Read the model definition and answer for the solid it produces. Units are mm, in the model's axes. Coordinates: 2 decimals unless noted, no trailing zeros. Order: outer loops, then holes, each group sorted by start corner. A loop starts at its lowest first (then second) coordinate and runs counter-clockwise, first axis right, second up. Notation, with made-up numbers: M 12,-25 L 22,-25 A26 cw 22,12 Z; hole C 68.5,36 d8. An arc over 180 degrees is marked long. Put each result on its own line as item: value.
from build123d import *

# Parameters (mm, degrees)
SKETCH1_R           = 13
BOSS_EXTRUDE1_DEPTH = 5.5
FILLET2_R           = 3


with BuildPart() as part:
    # Sketch1 → Boss-Extrude1 (new, symmetric)
    with BuildSketch(Plane.XY):
        with BuildLine():
            Line((-15, -9.949874371), (-15, -209.949874371))
            Line((-15, -209.949874371), (15, -209.949874371))
            Line((15, -209.949874371), (15, -9.949874371))
            ThreePointArc((15, -9.949874371), (0, 18), (-15, -9.949874371))
        make_face()
        Circle(SKETCH1_R, mode=Mode.SUBTRACT)
    extrude(amount=BOSS_EXTRUDE1_DEPTH, both=True)

    # Fillet2
    # the kernel refuses this fillet: 3 mm, written as the material it adds along each edge
    with BuildSketch(Plane(origin=(15, -9.949874371, 5.5), x_dir=(0.5340574779916704, 0.8454481712093158, 0), z_dir=(0, 0, -1))) as fillet2_piece_1:
        with BuildLine():
            CenterArc((0.869355329, 2.999254564), FILLET2_R, 237.719985552, 31.002719134)
            Line((-0.732817105, 0.46291005), (0, 0))
            ThreePointArc((0, 0), (0.401240921, 0.004472619), (0.802481842, 0))
        make_face()
    extrude(amount=11)
    with BuildSketch(Plane(origin=(-15, -9.949874371, 5.5), x_dir=(0, -1, 0), z_dir=(0, 0, -1))) as fillet2_piece_2:
        with BuildLine():
            CenterArc((0.866779455, 3), FILLET2_R, 238.997280866, 31.002719134)
            ThreePointArc((-0.678456806, 0.428571429), (-0.336839767, 0.218067082), (0, 0))
            Line((0, 0), (0.866779455, 0))
        make_face()
    extrude(amount=11)
    # the kernel refuses this fillet: 3 mm, written as the material it takes off along each edge
    with BuildSketch(Plane(origin=(0, 0, -5.5), x_dir=(1, 0, 0), z_dir=(0, -1, 0))) as fillet2_2_piece_1:
        with BuildLine():
            CenterArc((13 + FILLET2_R, FILLET2_R), FILLET2_R, 180, 90)
            Line((13, FILLET2_R), (13, 0))
            Line((13, 0), (13 + FILLET2_R, 0))
        make_face()
    revolve(axis=Axis((0, 0, -5.5), (0, 0, 1)), mode=Mode.SUBTRACT)
    with BuildSketch(Plane(origin=(0, 0, 5.5), x_dir=(1, 0, 0), z_dir=(0, -1, 0))) as fillet2_2_piece_2:
        with BuildLine():
            CenterArc((13 + FILLET2_R, -FILLET2_R), FILLET2_R, 90, 90)
            Line((13, -FILLET2_R), (13, 0))
            Line((13, 0), (13 + FILLET2_R, 0))
        make_face()
    revolve(axis=Axis((0, 0, 5.5), (0, 0, 1)), mode=Mode.SUBTRACT)
    with BuildSketch(Plane(origin=(-22.5, -209.949874371, 5.5), x_dir=(0, 1, 0), z_dir=(1, 0, 0)), Plane(origin=(-22.5, -209.949874371, -5.5), x_dir=(0, 0, 1), z_dir=(1, 0, 0))) as fillet2_2_piece_3:
        with BuildLine():
            CenterArc((FILLET2_R, -FILLET2_R), FILLET2_R, 90, 90)
            Line((0, -FILLET2_R), (0, 0))
            Line((0, 0), (FILLET2_R, 0))
        make_face()
    extrude(amount=45, mode=Mode.SUBTRACT)
    with BuildSketch(Plane(origin=(15, -209.949874371, -13), x_dir=(-1, 0, 0), z_dir=(0, 0, 1)), Plane(origin=(-15, -209.949874371, -13), x_dir=(0, 1, 0), z_dir=(0, 0, 1))) as fillet2_2_piece_4:
        with BuildLine():
            CenterArc((FILLET2_R, -FILLET2_R), FILLET2_R, 90, 90)
            Line((0, -FILLET2_R), (0, 0))
            Line((0, 0), (FILLET2_R, 0))
        make_face()
    extrude(amount=26, mode=Mode.SUBTRACT)
    # the kernel refuses this fillet: 3 mm, written as the material it takes off along each edge
    with BuildSketch(Plane(origin=(-12, -206.949874371, 2.5), x_dir=(0, 0, 1), z_dir=(-1, 0, 0))) as fillet2_3_piece_1_section:
        Polygon((0, 0), (FILLET2_R, 0), (FILLET2_R, -FILLET2_R), (0, -FILLET2_R), align=None)
    fillet2_3_piece_1 = extrude(amount=FILLET2_R, mode=Mode.PRIVATE)
    fillet2_3_piece_1 = fillet2_3_piece_1 - Plane(origin=(-12, -206.949874371, 2.5), x_dir=(0, 0.7071067811865475, -0.7071067811865475), z_dir=(-1, 0, 0)) * Sphere(FILLET2_R, mode=Mode.PRIVATE)
    add(fillet2_3_piece_1, mode=Mode.SUBTRACT)
    with BuildSketch(Plane(origin=(-12, -206.949874371, -2.5), x_dir=(0, 0, -1), z_dir=(-1, 0, 0))) as fillet2_3_piece_2_section:
        Polygon((0, 0), (FILLET2_R, 0), (FILLET2_R, FILLET2_R), (0, FILLET2_R), align=None)
    fillet2_3_piece_2 = extrude(amount=FILLET2_R, mode=Mode.PRIVATE)
    fillet2_3_piece_2 = fillet2_3_piece_2 - Plane(origin=(-12, -206.949874371, -2.5), x_dir=(0, 0.7071067811865475, 0.7071067811865475), z_dir=(-1, 0, 0)) * Sphere(FILLET2_R, mode=Mode.PRIVATE)
    add(fillet2_3_piece_2, mode=Mode.SUBTRACT)
    with BuildSketch(Plane(origin=(12, -206.949874371, -2.5), x_dir=(1, 0, 0), z_dir=(0, 0, -1))) as fillet2_3_piece_3_section:
        Polygon((0, 0), (FILLET2_R, 0), (FILLET2_R, FILLET2_R), (0, FILLET2_R), align=None)
    fillet2_3_piece_3 = extrude(amount=FILLET2_R, mode=Mode.PRIVATE)
    fillet2_3_piece_3 = fillet2_3_piece_3 - Plane(origin=(12, -206.949874371, -2.5), x_dir=(-0.7071067811865475, 0.7071067811865475, 0), z_dir=(0, 0, -1)) * Sphere(FILLET2_R, mode=Mode.PRIVATE)
    add(fillet2_3_piece_3, mode=Mode.SUBTRACT)
    with BuildSketch(Plane(origin=(12, -206.949874371, 2.5), x_dir=(1, 0, 0), z_dir=(0, 0, 1))) as fillet2_3_piece_4_section:
        Polygon((0, 0), (FILLET2_R, 0), (FILLET2_R, -FILLET2_R), (0, -FILLET2_R), align=None)
    fillet2_3_piece_4 = extrude(amount=FILLET2_R, mode=Mode.PRIVATE)
    fillet2_3_piece_4 = fillet2_3_piece_4 - Plane(origin=(12, -206.949874371, 2.5), x_dir=(-0.7071067811865475, 0.7071067811865475, 0), z_dir=(0, 0, 1)) * Sphere(FILLET2_R, mode=Mode.PRIVATE)
    add(fillet2_3_piece_4, mode=Mode.SUBTRACT)
    with BuildSketch(Plane(origin=(15, -206.949874371, 5.5), x_dir=(-1, 0, 0), z_dir=(0, 1, 0)), Plane(origin=(-15, -10.816653826, -5.5), x_dir=(0, 0, 1), z_dir=(0, -1, 0))) as fillet2_3_piece_5:
        with BuildLine():
            CenterArc((FILLET2_R, -FILLET2_R), FILLET2_R, 90, 90)
            Line((0, -FILLET2_R), (0, 0))
            Line((0, 0), (FILLET2_R, 0))
        make_face()
    extrude(amount=196.133220545, mode=Mode.SUBTRACT)
    with BuildSketch(Plane(origin=(0, 0, 5.5), x_dir=(0.8571428571428582, -0.5150787536377108, 0), z_dir=(-0.5150787536377108, -0.8571428571428582, 0))) as fillet2_3_piece_6:
        with BuildLine():
            CenterArc((18 - FILLET2_R, -FILLET2_R), FILLET2_R, 0, 90)
            Line((18, -FILLET2_R), (18, 0))
            Line((18, 0), (18 - FILLET2_R, 0))
        make_face()
    revolve(axis=Axis((0, 0, 5.5), (0, 0, 1)), revolution_arc=242.005438268, mode=Mode.SUBTRACT)
    with BuildSketch(Plane(origin=(15, -206.949874371, -5.5), x_dir=(-1, 0, 0), z_dir=(0, 1, 0)), Plane(origin=(-15, -10.816653826, 5.5), x_dir=(0, 0, -1), z_dir=(0, -1, 0))) as fillet2_3_piece_7:
        with BuildLine():
            CenterArc((FILLET2_R, FILLET2_R), FILLET2_R, 180, 90)
            Line((0, FILLET2_R), (0, 0))
            Line((0, 0), (FILLET2_R, 0))
        make_face()
    extrude(amount=196.133220545, mode=Mode.SUBTRACT)
    with BuildSketch(Plane(origin=(0, 0, -5.5), x_dir=(0.8571428571428582, -0.5150787536377108, 0), z_dir=(-0.5150787536377108, -0.8571428571428582, 0))) as fillet2_3_piece_8:
        with BuildLine():
            CenterArc((18 - FILLET2_R, FILLET2_R), FILLET2_R, 270, 90)
            Line((18, FILLET2_R), (18, 0))
            Line((18, 0), (18 - FILLET2_R, 0))
        make_face()
    revolve(axis=Axis((0, 0, -5.5), (0, 0, 1)), revolution_arc=242.005438268, mode=Mode.SUBTRACT)
    with BuildSketch(Plane(origin=(-18, -10.816653826, 5.5), x_dir=(1, 0, 0), z_dir=(0, -1, 0))) as fillet2_3_piece_9:
        with BuildLine():
            CenterArc((3 + FILLET2_R, -FILLET2_R), FILLET2_R, 90, 90)
            Line((3, -FILLET2_R), (3, 0))
            Line((3, 0), (3 + FILLET2_R, 0))
        make_face()
    revolve(axis=Axis((-18, -10.816653826, 5.5), (0, 0, 1)), revolution_arc=31.002719134, mode=Mode.SUBTRACT)
    with BuildSketch(Plane(origin=(18, -10.816653826, -5.5), x_dir=(-0.8571428571428581, 0.5150787536377112, 0), z_dir=(0.5150787536377112, 0.8571428571428581, 0))) as fillet2_3_piece_10:
        with BuildLine():
            CenterArc((3 + FILLET2_R, FILLET2_R), FILLET2_R, 180, 90)
            Line((3, FILLET2_R), (3, 0))
            Line((3, 0), (3 + FILLET2_R, 0))
        make_face()
    revolve(axis=Axis((18, -10.816653826, -5.5), (0, 0, 1)), revolution_arc=31.002719134, mode=Mode.SUBTRACT)
    with BuildSketch(Plane(origin=(-18, -10.816653826, -5.5), x_dir=(1, 0, 0), z_dir=(0, -1, 0))) as fillet2_3_piece_11:
        with BuildLine():
            CenterArc((3 + FILLET2_R, FILLET2_R), FILLET2_R, 180, 90)
            Line((3, FILLET2_R), (3, 0))
            Line((3, 0), (3 + FILLET2_R, 0))
        make_face()
    revolve(axis=Axis((-18, -10.816653826, -5.5), (0, 0, 1)), revolution_arc=31.002719134, mode=Mode.SUBTRACT)
    with BuildSketch(Plane(origin=(18, -10.816653826, 5.5), x_dir=(-0.8571428571428581, 0.5150787536377112, 0), z_dir=(0.5150787536377112, 0.8571428571428581, 0))) as fillet2_3_piece_12:
        with BuildLine():
            CenterArc((3 + FILLET2_R, -FILLET2_R), FILLET2_R, 90, 90)
            Line((3, -FILLET2_R), (3, 0))
            Line((3, 0), (3 + FILLET2_R, 0))
        make_face()
    revolve(axis=Axis((18, -10.816653826, 5.5), (0, 0, 1)), revolution_arc=31.002719134, mode=Mode.SUBTRACT)


solid = part.part
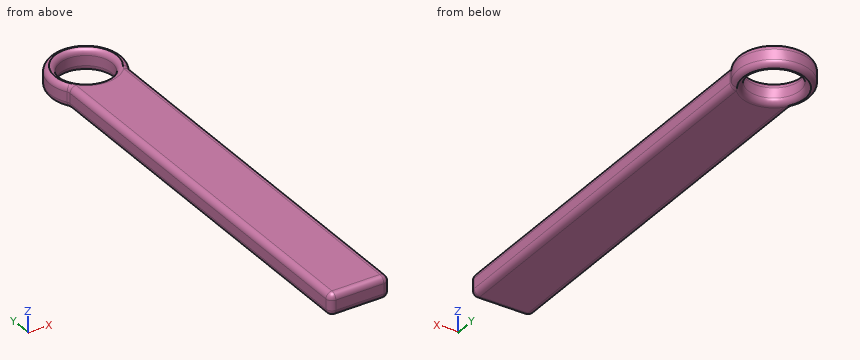
Q1. Find section B-B on y = 0. Write down the section's boundary in (x, z).
Answers below:
outline: M -18,-2.5 A3 ccw -15.5,-5.46 A3 ccw -13,-2.5 L -13,2.5 A3 ccw -15.5,5.46 A3 ccw -18,2.5 Z; M 13,-2.5 A3 ccw 15.5,-5.46 A3 ccw 18,-2.5 L 18,2.5 A3 ccw 15.5,5.46 A3 ccw 13,2.5 Z
Q2. Consider line 1 along Y through (x, z) = (0, -0.55); line 2 along Y through (x, z) = (10.5, -1.75); line 3 along X through (y, z) = (-57.5, -2.5). Determine where each line is inside the solid, lowest interval first.
Answers below:
line 1: y = -209.95 to -13, 13 to 18
line 2: y = -209.95 to -7.66, 7.66 to 14.62
line 3: x = -15 to 15
Q3. Find section A-A on x = 0. Write down the section's boundary in (y, z), plus the area to 3 significant figures.
Answers below:
outline: M -209.95,-2.5 A3 ccw -206.95,-5.5 L -16,-5.5 A3 ccw -13,-2.5 L -13,2.5 A3 ccw -16,5.5 L -206.95,5.5 A3 ccw -209.95,2.5 Z; M 13,-2.5 A3 ccw 15.5,-5.46 A3 ccw 18,-2.5 L 18,2.5 A3 ccw 15.5,5.46 A3 ccw 13,2.5 Z
area: 2,210 mm^2
Q4. Find section C-C on y = -80.5. Write down the section's boundary in (x, z), plus the area to 3 significant figures.
Answers below:
outline: M -15,-2.5 A3 ccw -12,-5.5 L 12,-5.5 A3 ccw 15,-2.5 L 15,2.5 A3 ccw 12,5.5 L -12,5.5 A3 ccw -15,2.5 Z
area: 322 mm^2
Q5. Given pin 1 (2 mm diameter, centred on x = -14, z = 1, fed in from -Y); pin 2 (1.5 mm diameter, centred on y = -95.5, z = -3.5, fed in from +X); pin 3 (6 mm diameter, centred on y = -39, z = 1, fed in from -X), each flat-ended and moving along its own axis, determine where each tip first touches the part or whether it passes through.
Answers below:
pin 1: stops at y = -209.78
pin 2: stops at x = 14.99
pin 3: stops at x = -15
